Geometry: final body of the model. Coordinates: model frame, mm. A direction names the side the tool comes from. Give positions to 0.01 mm unless a question says otherwise; leave off trailing zeros. Loops run counter-clockwise (first coordinate to the right, second up) from the corner with the lowest first, then second, coordinate; pieces in that order, holes last.
1. Draft query along X for faces 4 (the face through (4.28, 4.51, 1.05)), 5 (the face through (5, 5.2, 1)), 6 (the face through (142, 185, -75)). Return one class per face: +X half, -X half, draft (parallel to the pull), parting line (faces both ways), or undercut.
2. Section A-A, the plane y = 140. Output: boundary loops of the cut face in (x, z).
3. Access query for faces 1 (the face through (142, 185, 75)), 2 (the face through (288, 180, 1)), 3 (the face through (143, 1, 1)). Directions: +Z, -Z, +X, -X, +Y, -Y. A direction counts if a zero-diameter tool reaches every point of the face in a straight line with its end or side. Return the directions, or none.
4. Section B-B, the plane y = 303.1. Output: boundary loops of the cut face in (x, z), then the cut area to 3 significant figures.
5. First-contact query: P1, Ø6, axis at x = 155, z = -17.5, coming from the +Y side; P2, Ø1.4, axis at x = 89, y = 351.5, coming from the +Z side; P3, Ø5, axis at y = 285.5, z = -46, coming from the +X side. Flat tips, straight axial feed; report the tip coordinate or a pass-through.
6. Material intervals for line 1 along X through (y, z) = (123, 67.5); line 2 along Z through (x, y) = (234, 202.5); line 3 along Y through (x, z) = (191, 45.5), sorted ascending.
from build123d import *

# Parameters (mm, degrees)
SKETCH1_W           = 289
SKETCH1_H           = 350
BOSS_EXTRUDE1_DEPTH = 75
FILLET1_R           = 15
SHELL1_T            = -1
SKETCH5_R           = 18
CUT_EXTRUDE1_DEPTH  = 10
SKETCH6_R           = 17
CUT_EXTRUDE2_DEPTH  = 10


with BuildPart() as part:
    # Sketch1 → Boss-Extrude1 (new, symmetric)
    with BuildSketch(Plane.XY):
        with Locations((144.5, 175)):
            Rectangle(SKETCH1_W, SKETCH1_H)
    extrude(amount=BOSS_EXTRUDE1_DEPTH, both=True)

    # Fillet1
    fillet1_edges = [part.edges().sort_by_distance(p)[0] for p in [
        (144.5, 0, 75),
        (289, 0, 0),
        (0, 0, 0),
        (144.5, 0, -75),
    ]]
    fillet(fillet1_edges, radius=FILLET1_R)

    # Shell1
    shell1_openings = [part.faces().sort_by_distance(p)[0] for p in [
        (144.5, 350, 0),
    ]]
    offset(amount=SHELL1_T, openings=shell1_openings)

    # Sweep1: sweep along a path in Sketch3
    with BuildLine(Plane(origin=(0, 350, 0), x_dir=(1, 0, 0), z_dir=(0, 1, 0))) as sweep1_path:
        Line((288.5, -74.5), (288.5, 74.5))
        Line((288.5, 74.5), (0.5, 74.5))
        Line((0.5, 74.5), (0.5, -74.5))
        Line((0.5, -74.5), (288.5, -74.5))
    # Sketch4 → Sweep1 (sweep)
    with BuildSketch(Plane.XY):
        with BuildLine():
            Line((-0.65, 350), (1.65, 350))
            ThreePointArc((1.65, 350), (1.720710678, 350.029289322), (1.75, 350.1))
            Line((1.75, 350.1), (1.75, 350.4))
            ThreePointArc((1.75, 350.4), (1.720710678, 350.470710678), (1.65, 350.5))
            Line((1.65, 350.5), (0.85, 350.5))
            ThreePointArc((0.85, 350.5), (0.779289322, 350.529289322), (0.75, 350.6))
            Line((0.75, 350.6), (0.75, 351.9))
            ThreePointArc((0.75, 351.9), (0.720710678, 351.970710678), (0.65, 352))
            Line((0.65, 352), (0.35, 352))
            ThreePointArc((0.35, 352), (0.279289322, 351.970710678), (0.25, 351.9))
            Line((0.25, 351.9), (0.25, 350.6))
            ThreePointArc((0.25, 350.6), (0.220710678, 350.529289322), (0.15, 350.5))
            Line((0.15, 350.5), (-0.65, 350.5))
            ThreePointArc((-0.65, 350.5), (-0.720710678, 350.470710678), (-0.75, 350.4))
            Line((-0.75, 350.4), (-0.75, 350.1))
            ThreePointArc((-0.75, 350.1), (-0.720710678, 350.029289322), (-0.65, 350))
        make_face()
    sweep(path=sweep1_path.line, transition=Transition.RIGHT)

    # Sketch5 → Cut-Extrude1 (cut)
    with BuildSketch(Plane.XZ):
        with Locations(Location((243.128583469, 0, 0), (0, 0, 270))):
            Circle(SKETCH5_R)
    extrude(amount=-CUT_EXTRUDE1_DEPTH, mode=Mode.SUBTRACT)

    # Sketch6 → Cut-Extrude2 (cut)
    with BuildSketch(Plane.ZY):
        with Locations((-43, 303.1)):
            Circle(SKETCH6_R)
    extrude(amount=-CUT_EXTRUDE2_DEPTH, mode=Mode.SUBTRACT)


solid = part.part
Answers below:
1. face 4: -X half
1. face 5: undercut
1. face 6: draft
2. outline: (0, -75) - (289, -75) - (289, 75) - (0, 75) - close; hole (1, -74) - (288, -74) - (288, 74) - (1, 74) - close
3. face 1: +Z, +X, -X, -Y
3. face 2: none
3. face 3: +Y
4. outline: (0, -75) - (289, -75) - (289, 75) - (0, 75) - (0, -26) - (1, -26) - (1, 74) - (288, 74) - (288, -74) - (1, -74) - (1, -60) - (0, -60) - close
4. area: 840 mm2
5. P1: stops at y = 1
5. P2: stops at z = 74.75
5. P3: stops at x = 289
6. line 1: x = 0 to 1, 288 to 289
6. line 2: z = -75 to -74, 74 to 75
6. line 3: y = 0 to 1
